Verification items for the finished model (mm, model axes). A direction names the side the tool comes from. Coordinates: 2 decimals unless noted, no trailing zeros. Order: outer loops, then holes, each group sorted by start corner. A loop starts at its lowest first (then second) coordinate and runs counter-clockwise, first axis right, second up. Notation, with made-up numbers: M 32,58 L 82,58 A19 cw 82,66 Z; hole C 54.25,-34 d11. An arc over 180 degrees is marked long. Return JSON: item names as keys, results as strings.
```python
from build123d import *

# Parameters (mm, degrees)
F0_R      = 63.5
F1_DEPTH  = 12.7
F2_R      = 38.1
F3_DEPTH  = 57.15
F5_R      = 50.8
F6_DEPTH  = 12.7
F8_W      = 50.8
F8_H      = 50.8
F9_DEPTH  = 82.55
F10_R     = 5.08
F12_R     = 6.35
F13_DEPTH = 25.4


with BuildPart() as f1:
    # F0 (on Top) → F1 (new body)
    with BuildSketch(Plane.XY):
        Circle(F0_R)
    extrude(amount=F1_DEPTH)

    # F2 (on Top) → F3 (join)
    with BuildSketch(Plane.XY):
        Circle(F2_R)
    extrude(amount=F3_DEPTH)


with BuildPart() as f1_1:
    # F4: moved
    add(f1.part.moved(Location((0, 0, -57.1246))))

    # F5 (on Top) → F6 (join)
    with BuildSketch(Plane.XY):
        Circle(F5_R)
    extrude(amount=F6_DEPTH)


with BuildPart() as f1_2:
    # F7: moved
    add(f1_1.part.moved(Location((0, 0, -12.7))))

    # F8 (on Top) → F9 (cut)
    with BuildSketch(Plane.XY):
        Rectangle(F8_W, F8_H)
    extrude(amount=-F9_DEPTH, mode=Mode.SUBTRACT)

    # F10
    f10_edges = [f1_2.edges().sort_by_distance(p)[0] for p in [
        (-50.8, 0, 0),
    ]]
    fillet(f10_edges, radius=F10_R)


with BuildPart() as f1_3:
    # F11: moved
    add(f1_2.part.moved(Location((0, 0, 57.1246))))

    # F12 (on Top) → F13 (cut)
    with BuildSketch(Plane.XY):
        with Locations((0, -50.8)):
            Circle(F12_R)
        with Locations((50.8, 0)):
            Circle(F12_R)
        with Locations((0, 50.8)):
            Circle(F12_R)
        with Locations((-50.8, 0)):
            Circle(F12_R)
    extrude(amount=-F13_DEPTH, mode=Mode.SUBTRACT)


solid = f1_3.part
```
Q1. Cross-section at D-D, the plane x = 49. State how many separate pieces and enclosed holes the cut face has, and give its area (3 significant figures).
Values:
{"separate pieces": "3", "enclosed holes": "0", "area": "1,160 mm^2"}
Q2. Go/stop test with flat-tipped pins: pin 1 (3 mm diameter, centred on x = 23, y = 44.5, fed in from +Z); pin 2 (7.5 mm diameter, centred on x = 0, y = 50.8, fed in from -Z); pin 3 (8 mm diameter, centred on x = 12.5, z = 25, fed in from -Y); pin 4 (3 mm diameter, centred on y = -40.5, z = 25, fed in from -X). Record where each tip stops, or that it passes through.
Values:
{"pin 1": "z = 56.23", "pin 2": "z = 44.42", "pin 3": "y = -37.14", "pin 4": "through"}
Q3. Material ranges on line 1 along Y through (x, z) = (0, -5.75); line 2 along Z through (x, y) = (-36, -18.5); line 3 along Y through (x, z) = (3, -0.5), recorded low to high.
Values:
{"line 1": "-63.5 to -57.15, -44.45 to -25.4, 25.4 to 44.45, 57.15 to 63.5", "line 2": "-12.7 to 0, 44.42 to 57.12", "line 3": "-63.43 to -56.4, -45.2 to -25.4, 25.4 to 45.2, 56.4 to 63.43"}
Q4. Cross-section at B-B, the plane z = 48. Record the boundary of the cut face in (x, y).
Values:
{"outline": "C 0,0 d101.6; hole M -25.4,-25.4 L 25.4,-25.4 L 25.4,25.4 L -25.4,25.4 Z"}
Q5. Cross-section at C-C, the plane y = 55. Record the boundary of the cut face in (x, z), and give its area (3 significant figures).
Values:
{"outline": "M -31.74,-12.7 L -4.76,-12.7 L -4.76,0 L -31.74,0 Z; M 4.76,-12.7 L 31.74,-12.7 L 31.74,0 L 4.76,0 Z", "area": "685 mm^2"}
Q6. Draft check along X on faces 1 (the face through (25.4, 0, 23)), 2 (the face through (-13.77, -61.99, -6.44)), 3 (the face through (27.3, -27.3, 0)). Enter one of: pulls with the +X half, pulls with the -X half, needs draft (parallel to the pull), parting line crosses it, or undercut.
Values:
{"face 1": "undercut", "face 2": "parting line crosses it", "face 3": "needs draft"}
Q7. Tool access check on faces 4 (the face through (7, 38, 44.425)), 5 (the face through (-25.4, 0, 23)), 6 (the face through (-44.743, 1.907, -6.261)), 7 (the face through (-11.012, -49.592, 48.181)). Record the directions out of +Z, -Z, +X, -X, +Y, -Y that give a thin tool (end or side, any length) a straight path to the whole face; none if there is none.
Values:
{"face 4": "none", "face 5": "+Z, -Z", "face 6": "-Z", "face 7": "+Z"}
Q8. Cross-section at A-A, the plane z = -2.5. Record the boundary of the cut face in (x, y).
Values:
{"outline": "C 0,0 d127; hole C -50.8,0 d12.7; hole M -25.4,-25.4 L 25.4,-25.4 L 25.4,25.4 L -25.4,25.4 Z; hole C 0,-50.8 d12.7; hole C 0,50.8 d12.7; hole C 50.8,0 d12.7"}
